Could you check a few things on this model? Use its own coordinates, in mm. A direction names the side the tool comes from. Give positions to 0.01 mm unless a question says otherwise; leave off trailing zeros. Write each loop counter-clockwise with the first axis right and the second up, starting at its lowest first coordinate (ties: lowest second). Pieces come first, ordered by that corner, then holes. Notation, with made-up numbers: M 71,-8.75 L 90,-8.75 A15 cw 90,4.25 Z; hole C -19,-15.5 d1. An arc over 180 degrees is marked long. Use one line per item in the form item = value.
Autodesk Fusion 360 part; units mm, degrees
sketch "スケッチ1" plane through (0, 0, 0) normal (0, 0, 1) x (1, 0, 0)
  line L0 (-53, -15) -> (0, -15)
  circle A0 centre (0, 0) radius 15
  line L1 (12.2873, 8.6036) -> (0.8064, 25)
  circle A1 centre (0, 0) radius 10.5
  line L2 (-33, 10.25) -> (-8, 10.25)
  line L3 (-8, 10.25) -> (-8, -10.25)
  line L4 (-8, -10.25) -> (-33, -10.25)
  line L5 (-33, -10.25) -> (-33, 10.25)
  line L6 (-13, 35) -> (13, 35)
  line L7 (-53, -15) -> (-58, -10)
  line L8 (-58, -10) -> (-58, 10)
  line L9 (-54, 8) -> (-38, 8)
  line L10 (-38, 8) -> (-38, -8)
  line L11 (-38, -8) -> (-54, -8)
  line L12 (-54, -8) -> (-54, 8)
  line L13 (-23, 15) -> (-53, 15)
  line L14 (-53, 15) -> (-58, 10)
  line L15 (-11.5, 10) -> (-11.5, -10)
  line L16 (-11.5, -10) -> (-17.5, -10)
  line L17 (-17.5, -10) -> (-17.5, -9.3)
  line L18 (-17.5, -9.3) -> (-29.7, -9.3)
  line L19 (-29.7, -9.3) -> (-29.7, 9.3)
  line L20 (-29.7, 9.3) -> (-17.5, 9.3)
  line L21 (-17.5, 9.3) -> (-17.5, 10)
  line L22 (-17.5, 10) -> (-11.5, 10)
  line L23 (-8, 6.8007) -> (-11.5, 6.8007)
  line L24 (-8, -6.8007) -> (-11.5, -6.8007)
  line L25 (0.8064, 25) -> (0.8064, 31)
  line L26 (0.8064, 31) -> (18, 31)
  line L27 (18, 31) -> (18, 39)
  line L28 (18, 39) -> (-18, 39)
  line L29 (-18, 39) -> (-23, 34)
  line L30 (-23, 34) -> (-23, 15)
  point P0 (-8, 0)
  point P1 (-11.5, 0)
  point P2 (-29.7, 0)
  point P3 (18, 35)
  dimension "d1" = 30
  dimension "d2" = 55
  dimension "d3" = 53
  dimension "d6" = 21
  dimension "d7" = 8
  dimension "d8" = 25
  dimension "d9" = 20.5
  dimension "d28" = 26
  dimension "d35" = 5
  dimension "d36" = 5
  dimension "d42" = 16
  dimension "d43" = 4
  dimension "d45" = 2
  dimension "d55" = 2
  dimension "d57" = 12.2
  dimension "d58" = 18.6
  dimension "d59" = 20
  dimension "d60" = 11.5
  dimension "d61" = 6
  dimension "d64" = 25
  dimension "d65" = 6
  dimension "d66" = 8
  dimension "d67" = 18
  dimension "d68" = 5
  dimension "d69" = 16
  dimension "d71" = 5
  dimension "d72" = 5
  dimension "d74" = 5
  dimension "d75" = 5
  dimension "d76" = 5
extrude "押し出し1" add sketch "スケッチ1" along normal blind 4 contours L0 A0 L1 L2 L4 L5 L7 L8 L13 L14 L25 L26 L27 L28 L29 L30 | A0 A1 L2 L3 L4 | A0 L2 L4 L5 L15 L16 L17 L18 L19 L20 L21 L22 | A0 L3 L4 L15 L24 | A0 L2 L3 L15 L23
hole "穴1" at (-8, 10.25, 0) at (-8, -10.25, 0) at (-33, -10.25, 0) at (-33, 10.25, 0) direction (0, 0, 1) diameter 2.1 depth 10 tip angle 118
hole "穴3" at (-13, 35, 0) at (13, 35, 0) direction (0, 0, 1) diameter 3.2 depth 10 tip angle 118
fillet "フィレット3" radius 2 4 edges at (-54, 8, 2) (-54, -8, 2) (-38, -8, 2) (-38, 8, 2)
fillet "フィレット4" radius 1 10 edges at (-53, -15, 2) (-58, -10, 2) (-58, 10, 2) (-53, 15, 2) (-23, 34, 2) (-18, 39, 2) (18, 39, 2) (18, 31, 2) (0.8064, 25, 2) (0.8064, 31, 2)
fillet "フィレット5" radius 5 1 edges at (-23, 15, 2)
1) Thinking about a two-plate mould opening in X: for faces 1 (the flat face through (-20, 37, 2)), 2 (the flat face through (-21, 12, 0)), 3 (the flat face through (-46, -8, 2)), which applies, released by +X, released by -X, zero draft, split by the parting line, or undercut?
Checked values:
face_1 = released by -X
face_2 = zero draft
face_3 = undercut
2) I want a section at C-C, the plane z = 1.65. Count the separate pieces of the cut face and the enclosed holes in it, plus the area to 3 significant figures.
Checked values:
separate_pieces = 1
enclosed_holes = 8
area = 1,810 mm2
3) For faces 4 (the flat face through (-23, 27, 2)), 5 (the flat face through (6.716, 16.56, 1.972)), 6 (the cylindrical face through (-38.6, -7.43, 2.03)), which set-ups out of +Z, -Z, +X, -X, +Y, -Y let a thin tool reach every point of the face, with its end or its side?
Checked values:
face_4 = +Z, -Z, -X, +Y
face_5 = +Z, -Z, +X
face_6 = +Z, -Z
4) If I drill on L1, parallel to Y at x = -8, z = 3.05; L2, parallel to Y at x = -13, z = 2.8; L3, parallel to Y at x = -43, z = 0.45, over which ranges is the centre line in solid material (lowest first)?
Checked values:
L1 = -15 to -11.3, -9.2 to -6.8, 6.8 to 9.2, 11.3 to 39
L2 = -15 to -10, 10 to 33.4, 36.6 to 39
L3 = -15 to -8, 8 to 15
5) I want a section at B-B, the plane x = 7. Please give me the cut outline in (y, z).
Checked values:
outline = M -13.27,0 L -7.83,0 L -7.83,4 L -13.27,4 Z; M 7.83,0 L 16.15,0 L 16.15,4 L 7.83,4 Z; M 31,0 L 39,0 L 39,4 L 31,4 Z
6) For pin 1 Ø3 at (x, y) = (13, 35) entering from +Z; pin 2 Ø1.5 at (x, y) = (-13, 19.5) entering from -Z; pin 3 Ø2 at (x, z) = (-36.5, 2.5) entering from +Y; pin 4 Ø2 at (y, z) = (28.5, 1.5) entering from +X, each with a flat end and sliding along its axis, tell me the tip position at first contact or that it passes through.
Checked values:
pin_1 = through
pin_2 = 0
pin_3 = 15
pin_4 = 0.81
7) I want a section at A-A, the plane x = -13. Please give me the cut outline in (y, z), plus the area to 3 significant figures.
Checked values:
outline = M -15,0 L -10,0 L -10,4 L -15,4 Z; M 10,0 L 33.4,0 L 33.4,4 L 10,4 Z; M 36.6,0 L 39,0 L 39,4 L 36.6,4 Z
area = 123 mm2
